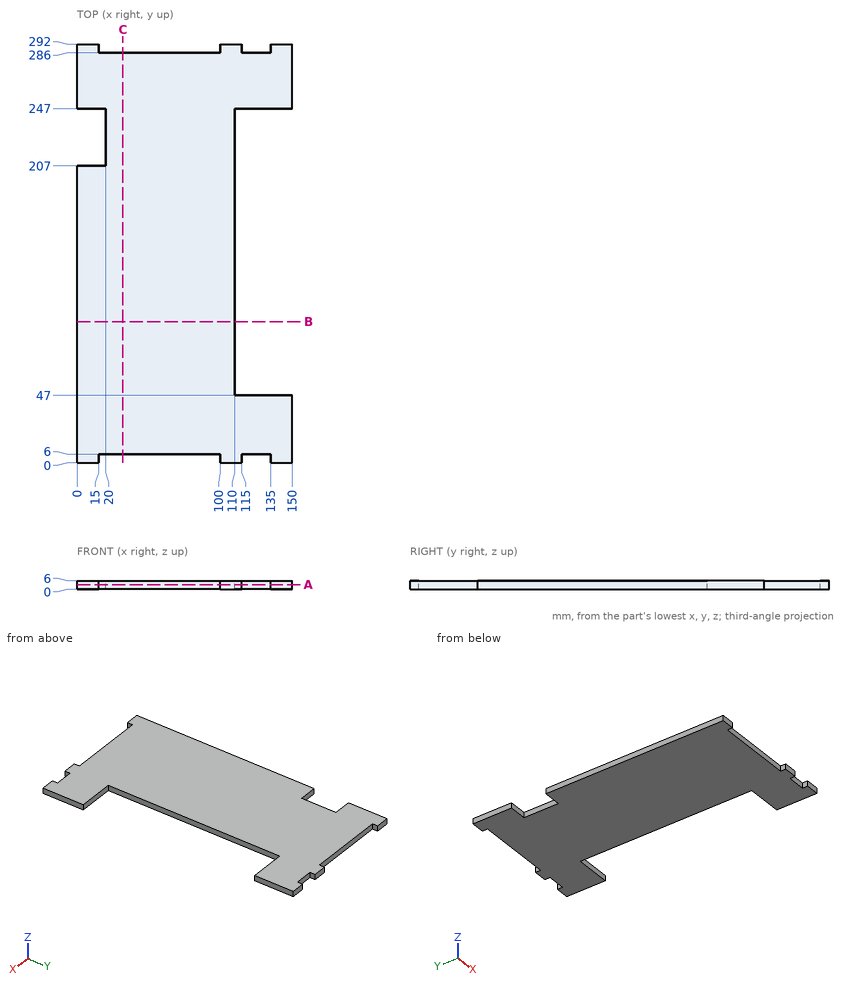
The drawing under review shows one solid part. Ordinate dimensions are in mm from its lowest x, y, z. Round coordinates to 2 decimals unless told otherwise and drop trailing zeros. Write each loop counter-clockwise with the first axis right and the second up, starting at its lowest first coordinate (ties: lowest second). Pieces come first, ordered by that corner, then holes. Notation, with made-up numbers: (32, 17) - (43, 17) arc R17 cw to (43, 27) - close; hole circle Ø5 at (70.5, -8). An arc over 180 degrees is marked (long way). Write each question's results on one line, items separated by ' | '.
Item 1: For pin 1 (1.8 mm diameter, centred on y = 289.5, z = 2.5, fed in from -X); pin 2 (4 mm diameter, centred on x = 113, y = 212.5, fed in from +Z); pin 3 (2 mm diameter, centred on x = 82, z = 5, fed in from +Y); pin 4 (1.8 mm diameter, centred on x = 68.5, z = 2.5, fed in from -Y), all flat-tipped, find the tip position at first contact; note any pin that passes through.
Calculated:
pin 1: stops at x = 0 | pin 2: passes through | pin 3: stops at y = 286 | pin 4: stops at y = 6
Item 2: Take a section at C-C on x = 32. State the section outline as (y, z) points.
Calculated:
outline: (6, 0) - (286, 0) - (286, 6) - (6, 6) - close
Item 3: Take a section at A-A on z = 3.35. State the section outline as (x, y) points, then the cut area to 3 significant figures.
Calculated:
outline: (0, 0) - (15, 0) - (15, 6) - (100, 6) - (100, 0) - (115, 0) - (115, 6) - (135, 6) - (135, 0) - (150, 0) - (150, 47) - (110, 47) - (110, 247) - (150, 247) - (150, 292) - (135, 292) - (135, 286) - (115, 286) - (115, 292) - (100, 292) - (100, 286) - (15, 286) - (15, 292) - (0, 292) - (0, 247) - (20, 247) - (20, 207) - (0, 207) - close | area: 33,700 mm^2
Item 4: Take a section at B-B on y = 98.5. State the section outline as (x, z) points, then the cut area to 3 significant figures.
Calculated:
outline: (0, 0) - (110, 0) - (110, 6) - (0, 6) - close | area: 660 mm^2
Item 5: To check wall thickness, follow line 1 along Y through (x, z) = (17.5, 2.4); line 2 along Y through (x, z) = (137, 1.8); line 3 along X through (y, z) = (66, 0.55). State the ranges of each line that lie inside material, in increasing order. Write a range as from..to.
Calculated:
line 1: y = 6..207, 247..286 | line 2: y = 0..47, 247..292 | line 3: x = 0..110
